Autodesk Inventor part; units mm, degrees
ref_plane "YZ Plane" through (0, 0, 0) normal (1, 0, 0) x (0, 1, 0)
ref_plane "XZ Plane" through (0, 0, 0) normal (0, 1, 0) x (-1, 0, 0)
ref_plane "XY Plane" through (0, 0, 0) normal (0, 0, 1) x (1, 0, 0)
sketch "スケッチ1" plane through (0, 0, 0) normal (1, 0, 0) x (0, 1, 0)
  circle A0 centre (0, 0) radius 9
  line L0 (9, 0) -> (-9, 0)
  line L1 (-9, 0) -> (-9, 25)
  line L2 (-9, 25) -> (9, 25)
  line L3 (9, 25) -> (9, 0)
  dimension "d0" = 18
  dimension "d1" = 25
  dimension "d2" = 18
extrude "押し出し1" add sketch "スケッチ1" along normal blind 3
sketch "スケッチ2" plane through (3, 0, 0) normal (1, 0, 0) x (0, 0, -1)
  line L0 (-25, 9) -> (-25, -9)
  line L1 (-25, -9) -> (-22, -9)
  line L2 (-22, -9) -> (-22, 9)
  line L3 (-22, 9) -> (-25, 9)
  line L4 (-25, 9) -> (-25, -9)
  line L5 (0, 9) -> (-25, 9)
  point P0 (0, 0)
  point P1 (-25, 9)
  dimension "d5" = 3
extrude "押し出し2" add sketch "スケッチ2" along normal blind 38.7
sketch "スケッチ3" plane through (41.7, 0, 0) normal (1, 0, 0) x (0, 0, -1)
  line L0 (-22, 9) -> (-22, -9)
  line L1 (-22, -9) -> (0, -9)
  arc A0 (0, -9) -> (0, 9) centre (0, 0) ccw
  line L2 (0, 9) -> (-22, 9)
  line L3 (-22, -9) -> (-22, 9)
  line L4 (-22, 9) -> (-25, 9)
  line L5 (-25, 9) -> (-25, -9)
  line L6 (-25, -9) -> (-22, -9)
extrude "押し出し3" add sketch "スケッチ3" along normal blind 3
sketch "スケッチ4" plane through (0, -9, 25) normal (0, 0, 1) x (1, 0, 0)
  line L0 (28.35, 22.75) -> (16.35, 22.75)
  line L1 (16.35, 22.75) -> (16.35, -4.75)
  line L2 (16.35, -4.75) -> (28.35, -4.75)
  line L3 (28.35, -4.75) -> (28.35, 22.75)
  line L4 (28.35, 22.75) -> (16.35, -4.75) construction
  line L5 (16.35, 22.75) -> (28.35, -4.75) construction
  line L6 (44.7, 18) -> (44.7, 0)
  line L7 (0, 0) -> (44.7, 0)
  line L8 (28.35, 15.75) -> (16.35, 15.75)
  point P0 (0, 9)
  point P1 (22.35, 9)
  dimension "d10" = 12
  dimension "d11" = 27.5
  dimension "d12" = 22.35
  dimension "d13" = 9
  dimension "d16" = 7
extrude "押し出し4" add sketch "スケッチ4" along normal blind 4.5 contours L3 L7 L1 L8 | L3 L2 L1 L7
sketch "スケッチ5" plane through (0, -9, 25) normal (0, 0, -1) x (-1, 0, 0)
  line L0 (-28.35, -4.75) -> (-28.35, 0)
  line L1 (-28.35, -4.75) -> (-16.35, -4.75)
  line L2 (-16.35, -4.75) -> (-16.35, -10.35)
  line L3 (-16.35, -10.35) -> (-28.35, -10.35)
  line L4 (-28.35, -10.35) -> (-28.35, -4.75)
  line L5 (-16.35, 15.75) -> (-16.35, -4.75)
  point P0 (0, 9)
  dimension "d17" = 5.6
extrude "押し出し5" add sketch "スケッチ5" against normal blind 32
sketch "スケッチ6" plane through (16.35, -13.75, 29.5) normal (0, 1, 0) x (1, 0, 0)
  line L0 (0, 0) -> (0, -27.5)
  line L1 (12, -27.5) -> (0, -27.5)
  line L2 (0, -27.5) -> (0, -23)
  line L3 (0, -23) -> (12, -23)
  line L4 (12, -23) -> (12, -27.5)
  line L5 (12, -27.5) -> (0, -27.5)
  line L6 (12, 0) -> (12, -27.5)
  point P0 (-16.35, 29.5)
  point P1 (6, -23)
  point P2 (0, -27.5)
  dimension "d20" = 4.5
extrude "押し出し6" add sketch "スケッチ6" along normal blind 20.5
sketch "スケッチ7" plane through (44.7, 0, 0) normal (1, 0, 0) x (0, 0, -1)
  circle A0 centre (0, 0) radius 6 construction
  line L0 (7.5318, 0) -> (-7.5318, 0) construction
  point P0 (-6, 0)
  point P1 (-4.2426, -4.2426)
  point P2 (0, -6)
  point P3 (4.2426, -4.2426)
  point P4 (6, 0)
  point P5 (4.2426, 4.2426)
  point P6 (0, 6)
  point P7 (-4.2426, 4.2426)
  dimension "d23" = 12
  dimension "d26" = 360
hole "穴1" at (44.7, 0, 6) at (44.7, -4.2426, 4.2426) at (44.7, -6, 0) at (44.7, -4.2426, -4.2426) at (44.7, 0, -6) at (44.7, 4.2426, -4.2426) at (44.7, 6, 0) at (44.7, 4.2426, 4.2426) direction (-1, 0, 0) diameter 2.4 depth 6.3
sketch "スケッチ8" plane through (16.35, -19.35, 25) normal (0, -1, 0) x (1, 0, 0)
  line L0 (0, 32) -> (12, 32) construction
  line L1 (6, 32) -> (6, 0) construction
  line L2 (0, 0) -> (12, 0) construction
  point P0 (-16.35, -25)
  point P1 (6, 21.79)
  dimension "d35" = 10.21
hole "穴2" at (22.35, -19.35, 46.79) direction (0, 1, 0) diameter 6.4 depth 6.3
sketch "スケッチ9" plane through (16.35, -19.35, 25) normal (0, -1, 0) x (1, 0, 0)
  circle A0 centre (6, 21.79) radius 3.2
  line L0 (12, 0) -> (0, 0)
  line L1 (12, 0) -> (12, 32)
  line L2 (0, 32) -> (12, 32)
  line L3 (0, 0) -> (0, 32)
  point P0 (-16.35, -25)
extrude "押し出し7" cut sketch "スケッチ9" against normal blind 1
sketch "スケッチ10" plane through (3, 0, 0) normal (1, 0, 0) x (0, 0, -1)
  circle A0 centre (0, 0) radius 3
  dimension "d45" = 6
extrude "押し出し8" add sketch "スケッチ10" along normal blind 5
sketch "スケッチ11" plane through (16.35, 6.75, 29.5) normal (0, 1, 0) x (1, 0, 0)
  circle A0 centre (6, -17.29) radius 3.2
  line L0 (6, -51.8359) -> (6, 17.2559)
  line L1 (37.0866, -11.5) -> (-25.0866, -11.5)
  line L2 (0, -27.5) -> (12, -27.5)
  line L3 (-16.35, 4.5) -> (28.35, 4.5)
  point P0 (-16.35, 29.5)
  point P1 (6, -11.5)
  point P2 (10, 2.5)
  point P3 (2, 2.5)
  point P4 (10, -25.5)
  point P5 (2, -25.5)
  dimension "d48" = 16
  dimension "d49" = 8
  dimension "d50" = 2
hole "穴3" at (26.35, 6.75, 27) at (18.35, 6.75, 27) at (26.35, 6.75, 55) at (18.35, 6.75, 55) direction (0, -1, 0) diameter 3 depth 3
chamfer "面取り1" distance 5 angle 45 2 edges at (41.7, 0, 22) (3, 0, 22)
chamfer "面取り2" distance 3 angle 45 2 edges at (22.35, -18.35, 57) (22.35, -18.35, 25)
chamfer "面取り3" distance 4.5 angle 45 2 edges at (16.35, -1.125, 25) (28.35, -1.125, 25)
chamfer "面取り4" distance 3 angle 45 3 edges at (22.35, -9, 25) (16.35, -9, 27.2499) (28.35, -9, 27.2499)
chamfer "面取り5" distance 3 angle 45 2 edges at (0, 0, 25) (44.7, 0, 25)
sketch "スケッチ12" plane through (0, -9, 57) normal (0, 0, 1) x (1, 0, 0)
  point P0 (0, 9)
sketch "スケッチ13" plane through (0, -9, 57) normal (0, 0, 1) x (1, 0, 0)
  line L0 (26.35, 6.25) -> (18.35, 6.25)
  line L1 (18.35, 6.25) -> (18.35, 0.25)
  line L2 (18.35, 0.25) -> (26.35, 0.25)
  line L3 (26.35, 0.25) -> (26.35, 6.25)
  line L4 (26.35, 6.25) -> (18.35, 0.25) construction
  line L5 (18.35, 6.25) -> (26.35, 0.25) construction
  line L6 (16.35, -4.75) -> (28.35, -4.75)
  line L7 (28.35, -6.35) -> (28.35, 15.75)
  point P0 (0, 9)
  point P1 (22.35, 3.25)
  dimension "d73" = 6
  dimension "d74" = 8
  dimension "d75" = 5
  dimension "d76" = 6
extrude "押し出し9" cut sketch "スケッチ13" against normal blind 10
sketch "スケッチ14" plane through (28.35, -13.75, 52.5) normal (1, 0, 0) x (0, 0, -1)
  line L0 (0, 11) -> (0, 5)
  line L1 (-4.5, 11) -> (0, 11)
  line L2 (-4.5, 5) -> (-4.5, 11)
  line L3 (-4.5, 5) -> (0, 5)
  line L4 (-2, 5) -> (-2, 11)
  point P0 (52.5, 13.75)
  dimension "d79" = 2
extrude "押し出し10" cut sketch "スケッチ14" against normal through all contours L0 L3 L4 L1
properties part number "Arm1"
The listing builds one solid part. Answer for the finished solid, in the listing's coordinates (mm). A direction names the side the tool comes from. Round coordinates to 2 decimals unless told otherwise and drop trailing zeros. Write each loop counter-clockwise with the first axis right and the second up, starting at its lowest first coordinate (ties: lowest second). Pieces come first, ordered by that corner, then holes. Notation, with made-up numbers: (54, 37) - (90, 37) arc R20 cw to (90, 50) - close; hole circle Ø7 at (35, -16). An arc over 180 degrees is marked (long way). Use a Markdown table: item, result. Add a question column.
1. Consider line 1 (Z direction, x = 18.35, y = 4.6); line 2 (X direction, y = 4.7, z = 55); line 3 (X direction, y = 5.5, z = 27). Determine where each line is inside the solid, lowest interval first.
2. Flat-ended cylindrical pins translate along their axes: P1, Ø3, axis at x = 20.5, y = 4, coming from the -Z side; P2, Ø2.5, axis at x = 23.5, y = -13, coming from the -Z side; P3, Ø2, axis at x = 25, z = 27.5, coming from the +Y side. Find the tip coordinate at first contact, or state that the pin passes through.
3. The part is cut by section A-A (z = 13). Write down the section's boundary in (x, y), and give its area (3 significant figures).
4. A tool of negligible diameter and unlimited length cuts with its end or side. For faces 4 (the face through (5, 0, 19)), 5 (the face through (43.179, -3.783, 3.134)), 6 (the face through (26.35, -6, 56)), from which of +Z, -Z, +X, -X, +Y, -Y can it reach the whole face along a straight path? Write none if from no direction.
5. For a pull along Y with two mould halves and no side action, classify faces 1 (the face through (43.18, -3.78, -5.35)), 2 (the face through (1, 0, -9)), 3 (the face through (14.83, -10.48, 25.8)) as +Y half, -Y half, draft (parallel to the pull), parting line (faces both ways), or undercut.
6. The part is cut by section B-B (x = 22.35). Give the number of separate pieces and of enclosed holes in the cut face, and give its area (3 significant figures).
7. The part is cut by section D-D (x = 6). Write down the section's boundary in (y, z).
Reported:
| question | item | result |
|---|---|---|
| 1 | line 1 | 22 to 25.5, 28.5 to 29.5, 52.5 to 53.5, 56.5 to 57 |
| 1 | line 2 | 16.35 to 16.85, 19.85 to 24.85, 27.85 to 28.35 |
| 1 | line 3 | 13.85 to 16.85, 19.85 to 24.85, 27.85 to 30.85 |
| 2 | P1 | z = 22 |
| 2 | P2 | z = 24.75 |
| 2 | P3 | y = 6.75 |
| 3 | outline | (0, -9) - (3, -9) - (3, 9) - (0, 9) - close; (41.7, -9) - (44.7, -9) - (44.7, 9) - (41.7, 9) - close |
| 3 | area | 108 mm^2 |
| 4 | face 4 | +Y, -Y |
| 4 | face 5 | +X |
| 4 | face 6 | +Z |
| 5 | face 1 | undercut |
| 5 | face 2 | parting line |
| 5 | face 3 | -Y half |
| 6 | separate pieces | 3 |
| 6 | enclosed holes | 0 |
| 6 | area | 325 mm^2 |
| 7 | outline | (-9, 20) - (9, 20) - (9, 25) - (-9, 25) - close; circle Ø6 at (0, 0) |
